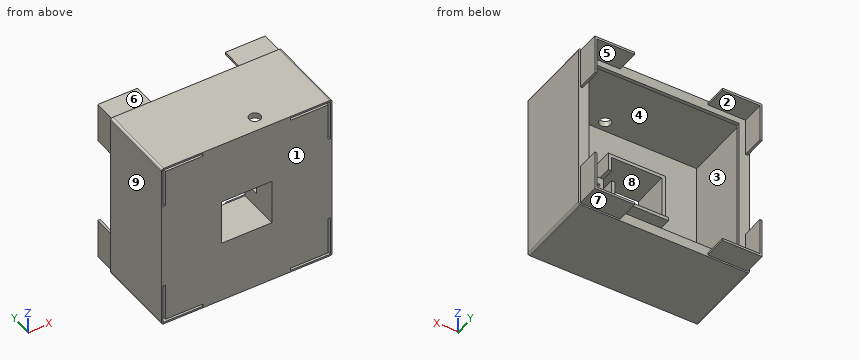
from build123d import *

# Parameters (mm, degrees)
SKETCH1_W           = 150
SKETCH1_H           = 150
BOSS_EXTRUDE1_DEPTH = 70
SHELL1_T            = -5
SKETCH2_W           = 50
SKETCH2_H           = 46
SKETCH2_W_2         = 44
SKETCH2_H_2         = 40
BOSS_EXTRUDE2_DEPTH = 32
CUT_EXTRUDE4_REACH  = 223.867
SKETCH5_W           = 44
SKETCH5_H           = 40
BOSS_EXTRUDE3_DEPTH = 20
SKETCH7_W           = 140
SKETCH7_H           = 140
SKETCH7_W_2         = 132
SKETCH7_H_2         = 132
BOSS_EXTRUDE4_DEPTH = 3
CUT_EXTRUDE5_REACH  = 203.494
SKETCH9_W           = 14
SKETCH9_H           = 15.8
SKETCH10_W          = 14
SKETCH10_H          = 3.5874966
BOSS_EXTRUDE5_DEPTH = 3.5
CUT_EXTRUDE6_REACH  = 225.01
SKETCH11_R          = 1.1
CUT_EXTRUDE8_DEPTH  = 4.5
FILLET1_R           = 2
CUT_EXTRUDE9_DEPTH  = 20.1
SKETCH14_R          = 5
CUT_EXTRUDE11_DEPTH = 20.1


with BuildPart() as part:
    # Sketch1 → Boss-Extrude1 (new body)
    with BuildSketch(Plane(origin=(0, 0, 0), x_dir=(1, 0, 0), z_dir=(0, 1, 0))):
        with Locations((75, 75)):
            Rectangle(SKETCH1_W, SKETCH1_H)
    extrude(amount=BOSS_EXTRUDE1_DEPTH)

    # Shell1
    shell1_openings = [part.faces().sort_by_distance(p)[0] for p in [
        (75, 70, -75),
    ]]
    offset(amount=SHELL1_T, openings=shell1_openings, kind=Kind.INTERSECTION)

    # Sketch2 → Boss-Extrude2 (add)
    with BuildSketch(Plane(origin=(0, 5, 0), x_dir=(1, 0, 0), z_dir=(0, 1, 0))):
        with Locations((75, 75.1)):
            Rectangle(SKETCH2_W, SKETCH2_H)
        with Locations((75, 75.1)):
            Rectangle(SKETCH2_W_2, SKETCH2_H_2, mode=Mode.SUBTRACT)
    extrude(amount=BOSS_EXTRUDE2_DEPTH)

    # Sketch5 → Cut-Extrude4 (cut, up to next)
    with BuildSketch(Plane(origin=(0, 5, 0), x_dir=(1, 0, 0), z_dir=(0, 1, 0)), mode=Mode.PRIVATE) as cut_extrude4_sk1:
        with Locations((75, 75.1)):
            Rectangle(SKETCH5_W, SKETCH5_H)
    cut_extrude4_tool1 = extrude(cut_extrude4_sk1.sketch, amount=-CUT_EXTRUDE4_REACH, mode=Mode.PRIVATE) & part.part
    add(cut_extrude4_tool1.solids().sort_by_distance((75, 5, -75.1))[0], mode=Mode.SUBTRACT)

    # Sketch6 → Boss-Extrude3 (add)
    with BuildSketch(Plane(origin=(0, 70, 0), x_dir=(1, 0, 0), z_dir=(0, 1, 0))):
        Polygon((1.5, 113.5), (1.5, 148.5), (36.5, 148.5), (36.5, 146.5), (3.5, 146.5), (3.5, 113.5), align=None)
        Polygon((1.5, 36.5), (1.5, 1.5), (36.5, 1.5), (36.5, 3.5), (3.5, 3.5), (3.5, 36.5), align=None)
        Polygon((148.5, 36.5), (148.5, 1.5), (113.5, 1.5), (113.5, 3.5), (146.5, 3.5), (146.5, 36.5), align=None)
        Polygon((148.5, 113.5), (148.5, 148.5), (113.5, 148.5), (113.5, 146.5), (146.5, 146.5), (146.5, 113.5), align=None)
    extrude(amount=BOSS_EXTRUDE3_DEPTH)

    # Sketch7 → Boss-Extrude4 (add)
    with BuildSketch(Plane(origin=(0, 70, 0), x_dir=(1, 0, 0), z_dir=(0, 1, 0))):
        with Locations((75, 75)):
            Rectangle(SKETCH7_W, SKETCH7_H)
        with Locations((75, 75)):
            Rectangle(SKETCH7_W_2, SKETCH7_H_2, mode=Mode.SUBTRACT)
    extrude(amount=-BOSS_EXTRUDE4_DEPTH)

    # Sketch9 → Cut-Extrude5 (cut, up to next)
    with BuildSketch(Plane(origin=(100, 0, 0), x_dir=(0, 0, -1), z_dir=(1, 0, 0)), mode=Mode.PRIVATE) as cut_extrude5_sk1:
        with Locations((75.1, 29.1)):
            Rectangle(SKETCH9_W, SKETCH9_H)
    cut_extrude5_tool1 = extrude(cut_extrude5_sk1.sketch, amount=-CUT_EXTRUDE5_REACH, mode=Mode.PRIVATE) & part.part
    add(cut_extrude5_tool1.solids().sort_by_distance((100, 29.1, -75.1))[0], mode=Mode.SUBTRACT)

    # Sketch10 → Boss-Extrude5 (add)
    with BuildSketch(Plane(origin=(100, 0, 0), x_dir=(0, 0, -1), z_dir=(1, 0, 0))):
        with Locations((75.1, 19.4062517)):
            Rectangle(SKETCH10_W, SKETCH10_H)
    extrude(amount=BOSS_EXTRUDE5_DEPTH)

    # Sketch11 → Cut-Extrude6 (cut, up to next)
    with BuildSketch(Plane(origin=(0, 21.2, 0), x_dir=(1, 0, 0), z_dir=(0, 1, 0)), mode=Mode.PRIVATE) as cut_extrude6_sk1:
        with Locations(Location((101.26, 75.55, 0), (0, 0, 270))):
            Circle(SKETCH11_R)
    cut_extrude6_tool1 = extrude(cut_extrude6_sk1.sketch, amount=-CUT_EXTRUDE6_REACH, mode=Mode.PRIVATE) & part.part
    add(cut_extrude6_tool1.solids().sort_by_distance((101.26, 21.2, -75.55))[0], mode=Mode.SUBTRACT)

    # Sketch12 → Cut-Extrude8 (cut)
    with BuildSketch(Plane(origin=(0, 37, 0), x_dir=(1, 0, 0), z_dir=(0, 1, 0))):
        Polygon((53, 95.1), (50, 95.1), (50, 52.1), (100, 52.1), (100, 68.1), (97, 68.1), (97, 55.1), (53, 55.1), align=None)
    extrude(amount=-CUT_EXTRUDE8_DEPTH, mode=Mode.SUBTRACT)

    # Fillet1
    fillet1_edges = [part.edges().sort_by_distance(p)[0] for p in [
        (0, 35, 0),
        (0, 35, -150),
        (150, 35, -150),
        (150, 35, 0),
    ]]
    fillet(fillet1_edges, radius=FILLET1_R)

    # Sketch13 → Cut-Extrude9 (cut)
    with BuildSketch(Plane.XZ):
        Polygon((1.5, -1.5), (36.6, -1.5), (36.6, -3.6), (3.6, -3.6), (3.6, -36.6), (1.5, -36.6), align=None)
        Polygon((148.5, -36.6), (148.5, -1.5), (113.4, -1.5), (113.4, -3.6), (146.4, -3.6), (146.4, -36.6), align=None)
        Polygon((148.5, -148.5), (113.4, -148.5), (113.4, -146.4), (146.4, -146.4), (146.4, -113.4), (148.5, -113.4), align=None)
        Polygon((1.5, -113.4), (1.5, -148.5), (36.6, -148.5), (36.6, -146.4), (3.6, -146.4), (3.6, -113.4), align=None)
    extrude(amount=-CUT_EXTRUDE9_DEPTH, mode=Mode.SUBTRACT)

    # Sketch14 → Cut-Extrude11 (cut)
    with BuildSketch(Plane(origin=(0, 0, -5), x_dir=(-1, 0, 0), z_dir=(0, 0, -1))):
        with Locations((-90.731434744, 13.61525696)):
            Circle(SKETCH14_R)
    extrude(amount=-CUT_EXTRUDE11_DEPTH, mode=Mode.SUBTRACT)


solid = part.part
Model file for the job. Use its own axes, mm. Face numbers are marked on the shaded views. A direction names the side the tool comes from. Round coordinates to 2 decimals unless told otherwise and drop trailing zeros. Order: outer loops, then holes, each group sorted by start corner. A loop starts at its lowest first (then second) coordinate and runs counter-clockwise, first axis right, second up.
(1) Pull direction Y, two halves, no side cores. Call the marked faces 1, 2, 3 and 4: released by +Y, released by -Y, zero draft, split by the parting line, or undercut.
(2) 3-axis set-ups, long thin cutter, end or side, ignore diameter. For the marked faces 5, 6, 7, 8 and 9: which of +Z, -Z, +X, -X, +Y, -Y reach the whole face in a straight line?
(3) Pin check, flat tips, straight feed: pin 1 (0.6 mm diameter, centred on y = 81, z = -147, fed in from +X); pin 2 (16 mm diameter, centred on y = 82.5, z = -27.5, fed in from -X); pin 3 (9 mm diameter, centred on x = 90.73, y = 13.62, fed in from +Z). Stop position of each tip, or through.
(4) Band-saw the part on C-C (y = 50). List the corners of the cut face in (x, z), then the cut area to 3 significant figures.
(5) Drill centre lines: line 1 (Z direction, x = 101, y = 19); line 2 (X direction, y = 18, z = -125.5); line 3 (X direction, y = 19.5, z = -86). Where is each one in solid material? Low to high.
(6) Band-saw the part on B-B (y = 27.5). List the corners of the cut face in (x, z), then the cut area to 3 significant figures.
(7) Band-saw the part on A-A (x = 78). List the corners of the cut face in (y, z).
(8) Band-saw the part on D-D (z = -138.5). List the corners of the cut face in (x, y).
Verdict:
1. face 1: released by -Y
1. face 2: zero draft
1. face 3: undercut
1. face 4: undercut
2. face 5: +Y
2. face 6: +Z, +X, -X, +Y
2. face 7: -Z, +X, -X, +Y
2. face 8: +Y, -Y
2. face 9: +Z, -Z, -X, +Y, -Y
3. pin 1: stops at x = 148.5
3. pin 2: stops at x = 1.5
3. pin 3: stops at z = -52.1
4. outline: (0, -148) arc R2 ccw to (2, -150) - (148, -150) arc R2 ccw to (150, -148) - (150, -2) arc R2 ccw to (148, 0) - (2, 0) arc R2 ccw to (0, -2) - close; hole (5, -145) - (145, -145) - (145, -5) - (5, -5) - close
4. area: 2,900 mm2
5. line 1: z = -150 to -145, -82.1 to -76.62, -74.48 to -68.1, -5 to 0
5. line 2: x = 0 to 1.5, 3.6 to 5, 145 to 146.4, 148.5 to 150
5. line 3: x = 0 to 5, 50 to 53, 97 to 100, 145 to 150
6. outline: (0, -148) arc R2 ccw to (2, -150) - (148, -150) arc R2 ccw to (150, -148) - (150, -2) arc R2 ccw to (148, 0) - (2, 0) arc R2 ccw to (0, -2) - close; (50, -98.1) - (100, -98.1) - (100, -82.1) - (97, -82.1) - (97, -95.1) - (53, -95.1) - (53, -55.1) - (97, -55.1) - (97, -68.1) - (100, -68.1) - (100, -52.1) - (50, -52.1) - close; hole (5, -145) - (145, -145) - (145, -5) - (5, -5) - close
6. area: 3,390 mm2
7. outline: (0, -150) - (70, -150) - (70, -141) - (67, -141) - (67, -145) - (5, -145) - (5, -98.1) - (37, -98.1) - (37, -95.1) - (0, -95.1) - close; (0, -55.1) - (32.5, -55.1) - (32.5, -52.1) - (5, -52.1) - (5, -5) - (67, -5) - (67, -9) - (70, -9) - (70, 0) - (0, 0) - close
8. outline: (0, 0) - (1.5, 0) - (1.5, 20.1) - (3.6, 20.1) - (3.6, 0) - (146.4, 0) - (146.4, 20.1) - (148.5, 20.1) - (148.5, 0) - (150, 0) - (150, 70) - (148.5, 70) - (148.5, 90) - (146.5, 90) - (146.5, 70) - (141, 70) - (141, 67) - (145, 67) - (145, 5) - (5, 5) - (5, 67) - (9, 67) - (9, 70) - (3.5, 70) - (3.5, 90) - (1.5, 90) - (1.5, 70) - (0, 70) - close
